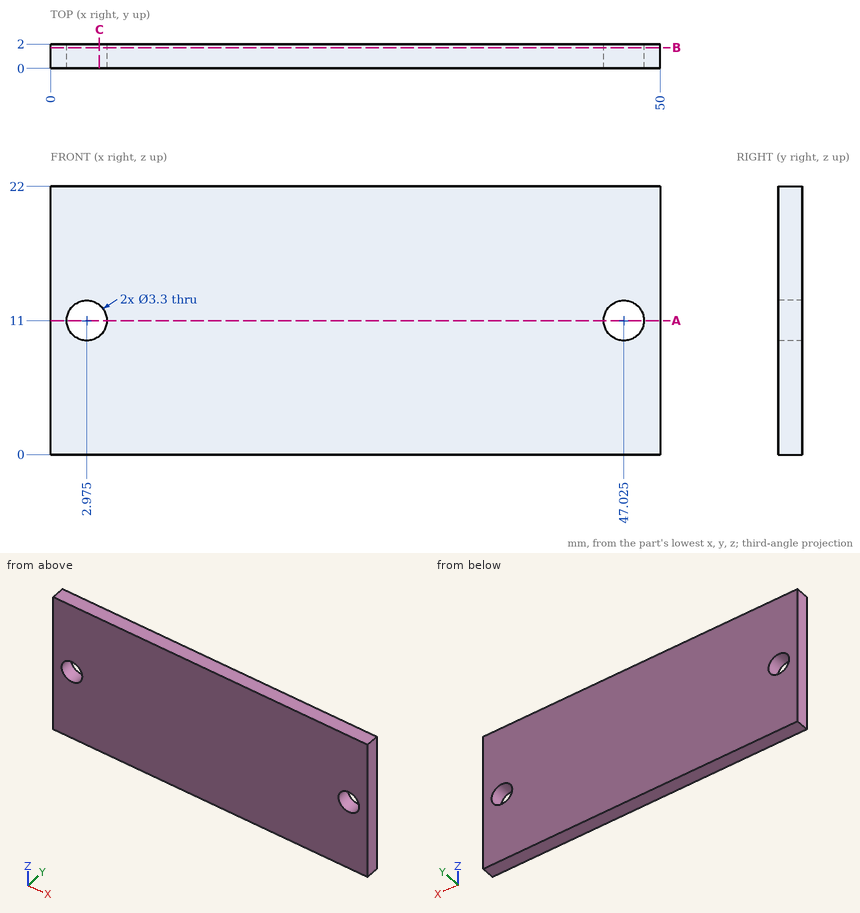
Check sheet for the drawn part. Datum: minimum x, y, z corner. Units: mm. Give positions to 0.01 mm unless a question says otherwise; leave off trailing zeros. Loops run counter-clockwise (first coordinate to the right, second up) from the corner with the lowest first, then second, coordinate; pieces in that order, holes last.
1) Sectioned sample at C-C, the plane x = 4. Enter the section's corners in (y, z).
2) Sectioned sample at B-B, the plane y = 1.7. Enter the section's corners in (x, z) (3 decimals).
3) Thickness scan on line 1 along Z through (x, y) = (47, 1.35); line 2 along Z through (x, y) = (48, 1.05). Record the ranges inside material, lowest first.
4) Sectioned sample at A-A, the plane z = 11. Enter the section's corners in (x, y) (3 decimals).
Answers:
1. outline: (0, 0) - (2, 0) - (2, 9.71) - (0, 9.71) - close; (0, 12.29) - (2, 12.29) - (2, 22) - (0, 22) - close
2. outline: (0, 0) - (50, 0) - (50, 22) - (0, 22) - close; hole circle Ø3.3 at (2.975, 11); hole circle Ø3.3 at (47.025, 11)
3. line 1: z = 0 to 9.35, 12.65 to 22
3. line 2: z = 0 to 9.67, 12.33 to 22
4. outline: (0, 0) - (1.325, 0) - (1.325, 2) - (0, 2) - close; (4.625, 0) - (45.375, 0) - (45.375, 2) - (4.625, 2) - close; (48.675, 0) - (50, 0) - (50, 2) - (48.675, 2) - close
